```python
from build123d import *

# Parameters (mm, degrees)
F1_DEPTH = 12.7
F2_T     = -3.175
F3_R     = 6.35
F5_W     = 12.7
F5_H     = 6.35
F6_DEPTH = 9.398


# Not quite as in the source:
# - a feature names something its author has since deleted; it is built from what else it names


with BuildPart() as f1:
    # F0 (on Top) → F1 (new body)
    with BuildSketch(Plane.XY):
        with BuildLine():
            Line((58.0965084505, 62.5356453779), (-58.0965084505, 62.5356453779))
            ThreePointArc((-58.0965084505, 62.5356453779), (-66.1787389595, 59.1878758868), (-69.5265084505, 51.1056453779))
            Line((-69.5265084505, 51.1056453779), (-69.5265084505, -27.1992570698))
            ThreePointArc((-69.5265084505, -27.1992570698), (-67.0115325937, -35.1957139026), (-60.3721316603, -40.3130159932))
            ThreePointArc((-60.3721316603, -40.3130159932), (0, -51.0474727306), (60.3721316603, -40.3130159932))
            ThreePointArc((60.3721316603, -40.3130159932), (67.0115325937, -35.1957139026), (69.5265084505, -27.1992570698))
            Line((69.5265084505, -27.1992570698), (69.5265084505, 51.1056453779))
            ThreePointArc((69.5265084505, 51.1056453779), (66.1787389595, 59.1878758868), (58.0965084505, 62.5356453779))
        make_face()
    extrude(amount=F1_DEPTH)

    # F2
    f2_openings = [f1.faces().sort_by_distance(p)[0] for p in [
        (0, 7.919531, 12.7),
    ]]
    offset(amount=F2_T, openings=f2_openings)

    # F3
    f3_edges = [f1.edges().sort_by_distance(p)[0] for p in [
        (69.526508, 11.953194, 0),
        (66.178739, 59.187876, 0),
        (0, 62.535645, 0),
        (-66.178739, 59.187876, 0),
        (-69.526508, 11.953194, 0),
        (-67.011533, -35.195714, 0),
        (0, -51.047473, 0),
        (67.011533, -35.195714, 0),
    ]]
    fillet(f3_edges, radius=F3_R)

    # F5 (on offset) → F6 (join)
    with BuildSketch(Plane.XY.offset(12.7)):
        with Locations((-53.0805146158, 57.0815077901)):
            Rectangle(F5_W, F5_H)
        with Locations((53.0805146158, 57.0815077901)):
            Rectangle(F5_W, F5_H)
        Polygon((-41.6677072644, -33.773638308), (-58.6946308613, -33.773638308), (-60.6418885291, -37.9110425711), (-53.9016760886, -40.266495198), (-41.6677072644, -43.4330925345), align=None)
        Polygon((60.6418885291, -37.9110425711), (58.6946308613, -33.773638308), (41.6677072644, -33.773638308), (41.6677072644, -43.4330925345), (53.9016760886, -40.266495198), align=None)
    extrude(amount=-F6_DEPTH)


solid = f1.part
```
Part model, mm, in its own coordinate system. A direction names the side the tool comes from. Coordinates: 2 decimals unless noted, no trailing zeros. Order: outer loops, then holes, each group sorted by start corner. A loop starts at its lowest first (then second) coordinate and runs counter-clockwise, first axis right, second up. Notation, with made-up numbers: (57, -29.75) - (87, -29.75) arc R32 cw to (87, 9.25) - close; hole circle Ø1 at (60.5, -11.75). An arc over 180 degrees is marked (long way). Return JSON: item names as keys, results as strings. Group by question number.
Item 1: Which spindle directions (+Z, -Z, +X, -X, +Y, -Y) get a long thin tool onto all of the face, cutting with end or side? Do faces 1 (the face through (-66.352, 13, 8)), 2 (the face through (66.267, 59.099, 9.481)). Say none if no direction does.
Item 2: Pin check, flat tips, straight feed: pin 1 (4.5 mm diameter, centred on y = -39, z = 9, fed in from -X); pin 2 (5 mm diameter, centred on x = -22.5, z = 7, fed in from -Y); pin 3 (1.5 mm diameter, centred on x = 54.5, z = 2, fed in from +Y). Stop position of each tip, or through.
Item 3: Drill centre lines: probe 1 along X at (y, z) = (-21, 11.75); probe 2 along Z at (x, y) = (5, -43) (3 decimals); probe 3 along Y at (x, z) = (-62, 4). Where is each one in solid material? Low to high. Write a range as from..to.
Item 4: Pull direction Y, two halves, no side cores. Call faces 3 (the face through (50, -33.774, 8)), 4 (the face through (-0.863, -51.045, 9.481)), 5 (the face through (1, 62.536, 9)): pulls with the +Y half, pulls with the -Y half, needs draft (parallel to the pull), parting line crosses it, or undercut.
Item 5: Cut at A-A (z = 10.25). List the corners of the cut face in (x, y) (1 decimal), plus the area to 3 significant figures.
Check values:
{
 "1": {"face 1": "+Z", "face 2": "+Z, -Z, +X, +Y"},
 "2": {"pin 1": "stops at x = -65.75", "pin 2": "stops at y = -49.9", "pin 3": "stops at y = 61.42"},
 "3": {"probe 1": "x = -69.53..-66.35, 66.35..69.53", "probe 2": "z = 0..3.175", "probe 3": "y = -39.08..-35.86, 58.38..61.37"},
 "4": {"face 3": "undercut", "face 4": "pulls with the -Y half", "face 5": "pulls with the +Y half"},
 "5": {"outline": "(-69.5, -27.2) arc R14 ccw to (-60.4, -40.3) arc R175.1 ccw to (60.4, -40.3) arc R14 ccw to (69.5, -27.2) - (69.5, 51.1) arc R11.4 ccw to (58.1, 62.5) - (-58.1, 62.5) arc R11.4 ccw to (-69.5, 51.1) - close; hole (-66.4, -27.2) arc R10.8 ccw to (-60.2, -36.9) - (-58.7, -33.8) - (-41.7, -33.8) - (-41.7, -42.7) arc R172 ccw to (41.7, -42.7) - (41.7, -33.8) - (58.7, -33.8) - (60.2, -36.9) arc R10.8 ccw to (66.4, -27.2) - (66.4, 51.1) arc R8.3 ccw to (59.4, 59.3) - (59.4, 53.9) - (46.7, 53.9) - (46.7, 59.4) - (-46.7, 59.4) - (-46.7, 53.9) - (-59.4, 53.9) - (-59.4, 59.3) arc R8.3 ccw to (-66.4, 51.1) - close", "area": "1,810 mm2"}
}
